```python
from build123d import *

# Parameters (mm, degrees)
F0_W        = 133.35
F0_H        = 50.8
F1_DEPTH    = 3.175
F2_W        = 19.05
F2_H        = 50.8
F3_DEPTH    = 38.1
F4_T        = 3.175
F4_T3_DEPTH = 57.15
F5_R        = 15.875
F7_DEPTH    = 25.4
F8_DEPTH    = 25.4
F9_R        = 1.5875
F10_DEPTH   = 25.4
F11_R       = 17.78


# Not quite as in the source:
# - a shell that OpenCascade refuses in one call is made with other operations: the cavity is built on its own and cut out


with BuildPart() as f1:
    # F0 (on Front) → F1 (new body)
    with BuildSketch(Plane.XZ):
        with Locations((66.675, 25.4)):
            Rectangle(F0_W, F0_H)
    extrude(amount=F1_DEPTH)

    # F2 (on face) → F3 (join)
    with BuildSketch(Plane.XZ.offset(3.175)):
        with Locations((9.525, 25.4)):
            Rectangle(F2_W, F2_H)
        with Locations((123.825, 25.4)):
            Rectangle(F2_W, F2_H)
    extrude(amount=F3_DEPTH)

    # F4: shell of thickness 3.175, made by hand


with BuildPart() as f4_core1:
    # F4_t2: copy of F1
    add(f1.part)

    # the walls: a layer under each face that stays
    f4_faces = [f4_core1.faces().sort_by_distance(p)[0] for p in [
        (0, -20.6375, 25.4),
        (66.675, 0, 25.4),
        (133.35, -20.6375, 25.4),
        (123.825, -41.275, 25.4),
        (114.3, -22.225, 25.4),
        (66.675, -3.175, 25.4),
        (19.05, -22.225, 25.4),
        (9.525, -41.275, 25.4),
        (123.825, -38.3267857143, 50.8),
    ]]
    thicken(f4_faces, amount=-F4_T, mode=Mode.SUBTRACT)

    # F4_s4 → F4_t3 (cut)
    with BuildSketch(Plane.XY.offset(-3.175)):
        Polygon((114.26825, -3.20675), (117.475, -3.175), (117.475, 0), (114.3, 0), align=None)
        Polygon((19.08175, -3.20675), (19.05, 0), (15.875, 0), (15.875, -3.175), align=None)
    extrude(amount=F4_T3_DEPTH, mode=Mode.SUBTRACT)


with BuildPart() as f1_1:
    add(f1.part)

    # what is left inside the walls is the cavity
    f4_cavity = [f4_core1.part.solids().sort_by_distance(p)[0] for p in [
        (3.20675, -26.458333, 23.8125),
        (130.14325, -26.458333, 23.8125),
    ]]
    add(f4_cavity, mode=Mode.SUBTRACT)

    # F5
    f5_edges = [f1_1.edges().sort_by_distance(p)[0] for p in [
        (9.525, -3.175, 47.625),
        (123.825, -3.175, 47.625),
        (9.525, -38.1, 47.625),
        (123.825, -38.1, 47.625),
    ]]
    fillet(f5_edges, radius=F5_R)

    # F6 (on face) → F7 (cut)
    with BuildSketch(Plane(origin=(15.875, 0, 0), x_dir=(0, -1, 0), z_dir=(-1, 0, 0))):
        with BuildLine():
            ThreePointArc((19.05, 47.625), (7.8246798487, 42.9753201513), (3.175, 31.75))
            Line((3.175, 31.75), (3.175, 0))
            Line((3.175, 0), (38.1, 0))
            Line((38.1, 0), (38.1, 31.75))
            ThreePointArc((38.1, 31.75), (33.4503201513, 42.9753201513), (22.225, 47.625))
            Line((22.225, 47.625), (19.05, 47.625))
        make_face()
    extrude(amount=-F7_DEPTH, mode=Mode.SUBTRACT)

    # F8 (cut): a face of the model
    f8_faces = [f1_1.faces().sort_by_distance(p)[0] for p in [
        (117.475, -20.6375, 22.4028811498),
    ]]
    extrude(f8_faces, amount=-F8_DEPTH, mode=Mode.SUBTRACT)

    # F9 (on face) → F10 (cut)
    with BuildSketch(Plane(origin=(0, 0, 0), x_dir=(-1, 0, 0), z_dir=(0, 1, 0))):
        with Locations((-47.625, 12.7)):
            Circle(F9_R)
        with Locations((-85.725, 12.7)):
            Circle(F9_R)
    extrude(amount=-F10_DEPTH, mode=Mode.SUBTRACT)

    # F11
    f11_edges = [f1_1.edges().sort_by_distance(p)[0] for p in [
        (9.525, -41.275, 50.8),
        (123.825, -41.275, 50.8),
    ]]
    fillet(f11_edges, radius=F11_R)


solid = f1_1.part
```
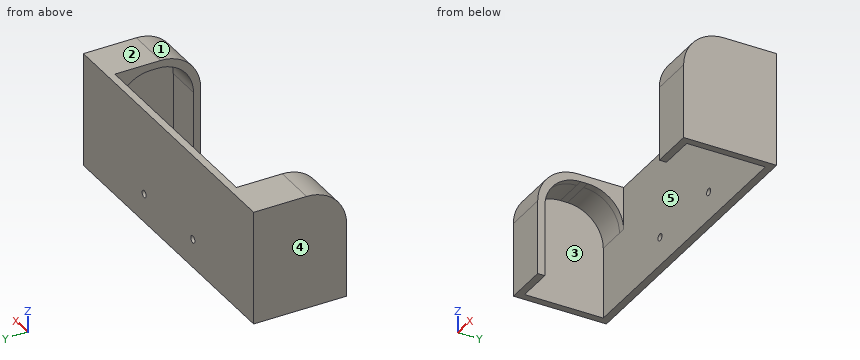
Geometry: final body of the model. Coordinates: model frame, mm. Face numbers are marked on the shaded views. A direction names the side the tool comes from. Round coordinates to 2 decimals unless told otherwise and drop trailing zeros. Order: outer loops, then holes, each group sorted by start corner. A loop starts at its lowest first (then second) coordinate and runs counter-clockwise, first axis right, second up. Notation, with made-up numbers: (11, 76) - (66, 76) arc R34 ccw to (66, 112) - close; hole circle Ø1 at (-8, 58.5). An arc over 180 degrees is marked (long way). Write item = value, one per line. Start each with the question number.
Q1. Cut plane A-A on y = -8. Return the cut outline in (x, z) (3 decimals), and give its area (3 significant figures).
Q2. Cut plane C-C on x = 123. Return the cut outline in (y, z) (3 decimals).
Q3. Ray query, line 1 (X direction, y = -33, z = 16) (3 decimals); line 2 (X direction, y = -3, z = 14); line 3 (Z direction, x = 119, y = -23). Return the intervals inside material, ascending. Write a range as from..to.
Q4. Cut plane D-D on z = 23. Return the cut outline in (x, y) (3 decimals).
Q5. Access query for the marked faces 4 and 5. Directions: +Z, -Z, +X, -X, +Y, -Y. A direction counts if a zero-diameter tool reaches every point of the face in a straight line with its end or side. Return the directions, or none.
Q6. Pin query (flat end, axial travel): pin 1 (2 mm diameter, centred on x = 65.5, z = 36.5, fed in from -Y) (3 decimals); pin 2 (1 mm diameter, centred on x = 11, y = -21.5, fed in from -Z) (3 decimals). Return the tip coordinate at first contact, or that it passes through.
Q7. Cut plane B-B on z = 12.7. Give the number of separate pieces and of enclosed holes in the cut face, and give its area (3 significant figures).
Q8. Pull-direction query (Y, two-part tool) for the marked faces 1, 2 and 3; classes: +Y half, -Y half, draft (parallel to the pull), parting line (faces both ways), or undercut.
Outcome:
q1.outline = (0, 0) - (3.175, 0) - (3.175, 43.148) - (19.05, 43.148) - (19.05, 50.8) - (0, 50.8) - close; (114.3, 43.148) - (130.175, 43.148) - (130.175, 0) - (133.35, 0) - (133.35, 50.8) - (114.3, 50.8) - close
q1.area = 566 mm^2
q2.outline = (-41.275, 0) - (-38.1, 0) - (-38.1, 31.75) arc R15.875 cw to (-22.225, 47.625) - (-19.05, 47.625) arc R15.875 cw to (-3.175, 31.75) - (-3.175, 0) - (0, 0) - (0, 50.8) - (-23.495, 50.8) arc R17.78 ccw to (-41.275, 33.02) - close
q3.line_1 = 0..3.175, 130.175..133.35
q3.line_2 = 0..46.71, 48.54..84.81, 86.64..133.35
q3.line_3 = 47.61..50.8
q4.outline = (0, -41.275) - (19.05, -41.275) - (19.05, -38.1) - (3.175, -38.1) - (3.175, -3.175) - (130.175, -3.175) - (130.175, -38.1) - (114.3, -38.1) - (114.3, -41.275) - (133.35, -41.275) - (133.35, 0) - (0, 0) - close
q5.face_4 = +Z, -Z, -X, +Y, -Y
q5.face_5 = -Z
q6.pin_1 = -3.175
q6.pin_2 = 47.625
q7.separate_pieces = 3
q7.enclosed_holes = 0
q7.area = 746 mm^2
q8.face_1 = -Y half
q8.face_2 = draft
q8.face_3 = undercut
